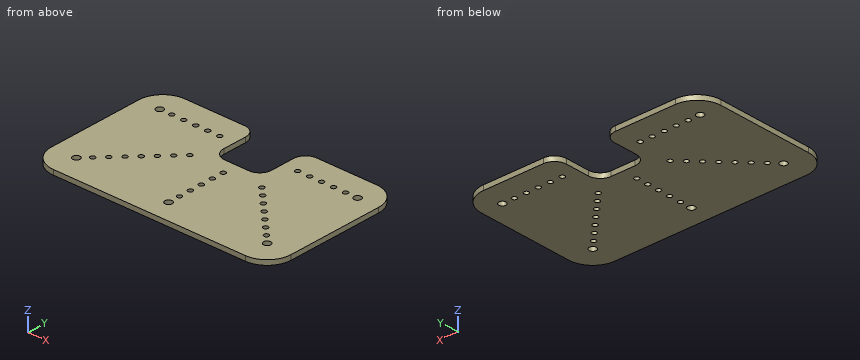
from build123d import *

# Parameters (mm, degrees)
SKETCH1_R           = 3
SKETCH1_R_2         = 2
BOSS_EXTRUDE1_DEPTH = 4
FILLET1_R           = 10
FILLET2_R           = 10
FILLET3_R           = 20


with BuildPart() as part:
    # Sketch1 → Boss-Extrude1 (new body)
    with BuildSketch(Plane.XY):
        Polygon((32.0494974, 36.578285273), (-47.9505026, 36.578285273), (-47.9505026, -3.421714727), (-87.9505026, -3.421714727), (-87.9505026, 36.578285273), (-167.9505026, 36.578285273), (-167.9505026, -83.421714727), (32.0494974, -83.421714727), align=None)
        with Locations((14.5494974, 16.578285273)):
            Circle(SKETCH1_R, mode=Mode.SUBTRACT)
        with Locations((-9.614193152, -41.758024175)):
            Circle(SKETCH1_R_2, mode=Mode.SUBTRACT)
        with Locations((-16.685260964, -34.686956363)):
            Circle(SKETCH1_R_2, mode=Mode.SUBTRACT)
        with Locations((-23.756328775, -27.615888551)):
            Circle(SKETCH1_R_2, mode=Mode.SUBTRACT)
        with Locations((-30.827396587, -20.544820739)):
            Circle(SKETCH1_R_2, mode=Mode.SUBTRACT)
        with Locations((-37.898464399, -13.473752928)):
            Circle(SKETCH1_R_2, mode=Mode.SUBTRACT)
        with Locations((-35.4505026, 16.578285273)):
            Circle(SKETCH1_R_2, mode=Mode.SUBTRACT)
        with Locations((-25.4505026, 16.578285273)):
            Circle(SKETCH1_R_2, mode=Mode.SUBTRACT)
        with Locations((-15.4505026, 16.578285273)):
            Circle(SKETCH1_R_2, mode=Mode.SUBTRACT)
        with Locations((-5.4505026, 16.578285273)):
            Circle(SKETCH1_R_2, mode=Mode.SUBTRACT)
        with Locations((4.5494974, 16.578285273)):
            Circle(SKETCH1_R_2, mode=Mode.SUBTRACT)
        with Locations((-2.54312534, -48.829091987)):
            Circle(SKETCH1_R_2, mode=Mode.SUBTRACT)
        with Locations((-67.9505026, -65.921714727)):
            Circle(SKETCH1_R, mode=Mode.SUBTRACT)
        with Locations((-67.9505026, -55.921714727)):
            Circle(SKETCH1_R_2, mode=Mode.SUBTRACT)
        with Locations((-67.9505026, -45.921714727)):
            Circle(SKETCH1_R_2, mode=Mode.SUBTRACT)
        with Locations((-67.9505026, -35.921714727)):
            Circle(SKETCH1_R_2, mode=Mode.SUBTRACT)
        with Locations((-67.9505026, -25.921714727)):
            Circle(SKETCH1_R_2, mode=Mode.SUBTRACT)
        with Locations((-67.9505026, -15.921714727)):
            Circle(SKETCH1_R_2, mode=Mode.SUBTRACT)
        with Locations((4.527942472, -55.900159799)):
            Circle(SKETCH1_R_2, mode=Mode.SUBTRACT)
        with Locations((-126.286812048, -41.758024175)):
            Circle(SKETCH1_R_2, mode=Mode.SUBTRACT)
        with Locations((-119.215744236, -34.686956363)):
            Circle(SKETCH1_R_2, mode=Mode.SUBTRACT)
        with Locations((-112.144676424, -27.615888551)):
            Circle(SKETCH1_R_2, mode=Mode.SUBTRACT)
        with Locations((-105.073608612, -20.544820739)):
            Circle(SKETCH1_R_2, mode=Mode.SUBTRACT)
        with Locations((-98.0025408, -13.473752928)):
            Circle(SKETCH1_R_2, mode=Mode.SUBTRACT)
        with Locations((11.599010284, -62.971227611)):
            Circle(SKETCH1_R, mode=Mode.SUBTRACT)
        with Locations((-150.4505026, 16.578285273)):
            Circle(SKETCH1_R, mode=Mode.SUBTRACT)
        with Locations((-140.4505026, 16.578285273)):
            Circle(SKETCH1_R_2, mode=Mode.SUBTRACT)
        with Locations((-130.4505026, 16.578285273)):
            Circle(SKETCH1_R_2, mode=Mode.SUBTRACT)
        with Locations((-120.4505026, 16.578285273)):
            Circle(SKETCH1_R_2, mode=Mode.SUBTRACT)
        with Locations((-110.4505026, 16.578285273)):
            Circle(SKETCH1_R_2, mode=Mode.SUBTRACT)
        with Locations((-100.4505026, 16.578285273)):
            Circle(SKETCH1_R_2, mode=Mode.SUBTRACT)
        with Locations((-133.357879859, -48.829091987)):
            Circle(SKETCH1_R_2, mode=Mode.SUBTRACT)
        with Locations((-140.428947671, -55.900159799)):
            Circle(SKETCH1_R_2, mode=Mode.SUBTRACT)
        with Locations((-147.500015483, -62.971227611)):
            Circle(SKETCH1_R, mode=Mode.SUBTRACT)
    extrude(amount=BOSS_EXTRUDE1_DEPTH)

    # Fillet1
    fillet1_edges = [part.edges().sort_by_distance(p)[0] for p in [
        (-87.9505026, -3.421714727, 2),
        (-47.9505026, -3.421714727, 2),
    ]]
    fillet(fillet1_edges, radius=FILLET1_R)

    # Fillet2
    fillet2_edges = [part.edges().sort_by_distance(p)[0] for p in [
        (-47.9505026, 36.578285273, 2),
        (-87.9505026, 36.578285273, 2),
    ]]
    fillet(fillet2_edges, radius=FILLET2_R)

    # Fillet3
    fillet3_edges = [part.edges().sort_by_distance(p)[0] for p in [
        (32.0494974, 36.578285273, 2),
        (32.0494974, -83.421714727, 2),
        (-167.9505026, -83.421714727, 2),
        (-167.9505026, 36.578285273, 2),
    ]]
    fillet(fillet3_edges, radius=FILLET3_R)


solid = part.part
For this review, take the finished solid that the model builds, in its own axes (mm). Round coordinates to 2 decimals unless told otherwise and drop trailing zeros. Write each loop counter-clockwise with the first axis right and the second up, starting at its lowest first coordinate (ties: lowest second). Pieces come first, ordered by that corner, then holes. Notation, with made-up numbers: (8.5, -15) - (24.5, -15) arc R31 cw to (24.5, 13) - close; hole circle Ø6 at (-17.5, 47.5). An arc over 180 degrees is marked (long way). Use a Markdown table: item, result.
Q1. We need section B-B (z = 3.3). State how many separate pieces and enclosed holes the cut face has, plus the area to 3 significant figures.
Derived:
| item | result |
|---|---|
| separate pieces | 1 |
| enclosed holes | 34 |
| area | 21,600 mm2 |
Q2. Clearance check with a flat-ended pin moving along its axis: pin 1 (1.2 mm diameter, centred on y = 18.5, z = 2.5, fed in from +X). State where the tip first meets the part, or that it passes through.
Derived:
| item | result |
|---|---|
| pin 1 | stops at x = 32.01 |
Q3. We need section A-A (y = 23.5). Give the boundary of the cut face in (x, z), plus the area to 3 significant figures.
Derived:
| item | result |
|---|---|
| outline | (-166.71, 0) - (-87.95, 0) - (-87.95, 4) - (-166.71, 4) - close; (-47.95, 0) - (30.81, 0) - (30.81, 4) - (-47.95, 4) - close |
| area | 630 mm2 |
Q4. Wall thickness on line 1 along Y through (x, z) = (-99, 0.25); line 2 along Y through (x, z) = (12, 1.9); line 3 along X through (y, z) = (-33, 1.7): over which ranges is each line inside the solid? List them lowest first.
Derived:
| item | result |
|---|---|
| line 1 | y = -83.42 to -15.21, -11.74 to 15.2, 17.96 to 36.58 |
| line 2 | y = -83.42 to -65.94, -60 to 15, 18.16 to 36.58 |
| line 3 | x = -167.95 to -120.29, -118.14 to -17.76, -15.61 to 32.05 |
Q5. We need section C-C (y = 1). Give the boundary of the cut face in (x, z).
Derived:
| item | result |
|---|---|
| outline | (-167.95, 0) - (-86.25, 0) - (-86.25, 4) - (-167.95, 4) - close; (-49.65, 0) - (32.05, 0) - (32.05, 4) - (-49.65, 4) - close |
Q6. We need section D-D (x = 20.5). Give the boundary of the cut face in (y, z).
Derived:
| item | result |
|---|---|
| outline | (-81.55, 0) - (34.71, 0) - (34.71, 4) - (-81.55, 4) - close |
